from build123d import *

# Parameters (mm, degrees)
AXIAL_PROFILE_MM_W     = 5
AXIAL_PROFILE_MM_H     = 34.4
AXIAL_HOLES_DEPTH      = 176.574514096
AXIAL_HOLES_DEPTH_BACK = 176.574514096
SKETCH2_R              = 1.65
CUT_EXTRUDE2_START     = 165.2
SKETCH3_R              = 1.65
CUT_EXTRUDE2_DEPTH     = 3.5


with BuildPart() as part:
    # Axial profile (mm) → Full revolution (revolve)
    with BuildSketch(Plane.XY, mode=Mode.PRIVATE) as full_revolution_sk:
        with Locations((166.2, 17.2)):
            Rectangle(AXIAL_PROFILE_MM_W, AXIAL_PROFILE_MM_H)
    revolve(full_revolution_sk.sketch.rotate(Axis((-110, 0, 0), (1, 0, 0)), 90), axis=Axis((-110, 0, 0), (1, 0, 0)))

    # Sketch2 → Axial holes (cut, two sides: drawn at the far end of the back side and taken through both)
    with BuildSketch(Plane(origin=(0, 0, 0), x_dir=(0, 0, -1), z_dir=(1, 0, 0)).offset(-AXIAL_HOLES_DEPTH_BACK)):
        with Locations((-29.4, 0)):
            Circle(SKETCH2_R)
        with Locations((14.7, -25.461146871)):
            Circle(SKETCH2_R)
        with Locations((14.7, 25.461146871)):
            Circle(SKETCH2_R)
    extrude(amount=AXIAL_HOLES_DEPTH + AXIAL_HOLES_DEPTH_BACK, mode=Mode.SUBTRACT)

    # Sketch3 → Cut-Extrude2 (cut)
    with BuildSketch(Plane(origin=(0, 0, 0), x_dir=(0, 0, -1), z_dir=(1, 0, 0)).offset(CUT_EXTRUDE2_START)):
        with Locations((29.4, 0)):
            Circle(SKETCH3_R)
        with Locations((-14.7, 25.461146871)):
            Circle(SKETCH3_R)
        with Locations((-14.7, -25.461146871)):
            Circle(SKETCH3_R)
    extrude(amount=-CUT_EXTRUDE2_DEPTH, mode=Mode.SUBTRACT)


solid = part.part
Here's how the part is built. I have some questions about the finished solid (model axes, mm). A direction names the side the tool comes from. Coordinates: 2 decimals unless noted, no trailing zeros. Order: outer loops, then holes, each group sorted by start corner. A loop starts at its lowest first (then second) coordinate and runs counter-clockwise, first axis right, second up. Notation, with made-up numbers: (39.5, 0.25) -> (74.5, 0.25) arc R10 cw to (74.5, 12.25) -> close; hole circle Ø6 at (10, 74). An arc over 180 degrees is marked (long way). Answer in a Markdown table with one row per item.
(1) I want a section at D-D on z = -30. List the corners of the cut face in (x, y) for me, then the cut area to 3 significant figures.
Answer key:
| item | result |
|---|---|
| outline | (163.7, -16.83) -> (168.7, -16.83) -> (168.7, 16.83) -> (163.7, 16.83) -> (163.7, 1.54) -> (165.2, 1.54) -> (165.2, -1.54) -> (163.7, -1.54) -> close |
| area | 164 mm^2 |
(2) I want a section at A-A on y = 0. List the corners of the cut face in (x, z) for me, then the cut area to 3 significant figures.
Answer key:
| item | result |
|---|---|
| outline | (163.7, -34.4) -> (168.7, -34.4) -> (168.7, 27.75) -> (163.7, 27.75) -> (163.7, -27.75) -> (165.2, -27.75) -> (165.2, -31.05) -> (163.7, -31.05) -> close; (163.7, 31.05) -> (168.7, 31.05) -> (168.7, 34.4) -> (163.7, 34.4) -> close |
| area | 323 mm^2 |
(3) On a 3-axis mill with a long thin cutter (end or side, diameter ignored), from which of +Z, -Z, +X, -X, +Y, -Y can I reach the whole of each face in a straight line? I mean faces 1 (the face through (163.7, 0, 0)), 2 (the face through (165.2, 0, -29)). Say none if no direction works.
Answer key:
| item | result |
|---|---|
| face 1 | +Z, -Z, -X, +Y, -Y |
| face 2 | -X |
(4) I want a section at B-B on z = 29. List the corners of the cut face in (x, y) for me.
Answer key:
| item | result |
|---|---|
| outline | (163.7, -18.5) -> (168.7, -18.5) -> (168.7, -1.6) -> (163.7, -1.6) -> close; (163.7, 1.6) -> (168.7, 1.6) -> (168.7, 18.5) -> (163.7, 18.5) -> close |
(5) Thinking about a two-plate mould opening in Y: for faces 3 (the face through (166.235, -1.513, -34.367)), 4 (the face through (168.7, 0, 0)), 5 (the face through (166.16, -24.07, -15.59)), which applies, +Y half, -Y half, draft (parallel to the pull), parting line (faces both ways), or undercut?
Answer key:
| item | result |
|---|---|
| face 3 | parting line |
| face 4 | draft |
| face 5 | undercut |
(6) Please list where these lines run through material, in increasing order: probe 1 along Z at (x, y) = (165.1, 1.5); probe 2 along Z at (x, y) = (164.8, -24.5); probe 3 along Y at (x, z) = (165.75, 28).
Answer key:
| item | result |
|---|---|
| probe 1 | -34.37 to -30.09, -28.71 to 28.71, 30.09 to 34.37 |
| probe 2 | -24.15 to -16.04, -13.36 to 13.36, 16.04 to 24.15 |
| probe 3 | -19.98 to -0.87, 0.87 to 19.98 |
(7) I want a section at C-C on z = -14.5. List the corners of the cut face in (x, y) for me, then the cut area to 3 significant figures.
Answer key:
| item | result |
|---|---|
| outline | (163.7, -31.19) -> (168.7, -31.19) -> (168.7, -27.1) -> (163.7, -27.1) -> close; (163.7, -23.82) -> (168.7, -23.82) -> (168.7, 23.82) -> (163.7, 23.82) -> close; (163.7, 27.1) -> (168.7, 27.1) -> (168.7, 31.19) -> (163.7, 31.19) -> close |
| area | 279 mm^2 |
(8) Will these pins go through, and if not, where does the flat tip stop? pin 1 Ø2 at (x, z) = (166.5, -20.5) entering from -Y; pin 2 Ø2.5 at (y, z) = (-25.5, 15) entering from -X; pin 3 Ø4 at (y, z) = (-25.46, -14.7) entering from +X; pin 4 Ø2 at (x, y) = (167, -23) entering from +Z.
Answer key:
| item | result |
|---|---|
| pin 1 | y = -28.34 |
| pin 2 | x = 165.2 |
| pin 3 | x = 168.7 |
| pin 4 | z = 26.45 |
